from build123d import *

# Parameters (mm, degrees)
CYLINDER002_R     = 0.95
CYLINDER002_DEPTH = 10
CYLINDER003_R     = 0.95
CYLINDER003_DEPTH = 10
CYLINDER_R        = 0.95
CYLINDER_DEPTH    = 10
CYLINDER001_R     = 0.95
CYLINDER001_DEPTH = 10
BOX_W             = 10
BOX_H             = 10
BOX_DEPTH         = 7
PAD_DEPTH         = 21


with BuildPart() as cylinder002:
    # Cylinder002 → Cylinder002 (new body)
    with BuildSketch(Plane(origin=(9.9, 0, 0), x_dir=(1, 0, 0), z_dir=(0, 0, 1))):
        Circle(CYLINDER002_R)
    extrude(amount=CYLINDER002_DEPTH)


with BuildPart() as tornillos001:
    # Cylinder003 → Cylinder003 (new body)
    with BuildSketch(Plane.XY):
        Circle(CYLINDER003_R)
    extrude(amount=CYLINDER003_DEPTH)

    # Fusion001: union Cylinder002
    add(cylinder002.part)


with BuildPart() as tornillos001_1:
    # Fusion001 placement: moved
    add(tornillos001.part.moved(Location((5, -24.5, 22))))


with BuildPart() as cylinder:
    # Cylinder → Cylinder (new body)
    with BuildSketch(Plane(origin=(9.9, 0, 0), x_dir=(1, 0, 0), z_dir=(0, 0, 1))):
        Circle(CYLINDER_R)
    extrude(amount=CYLINDER_DEPTH)


with BuildPart() as fusion002:
    # Cylinder001 → Cylinder001 (new body)
    with BuildSketch(Plane.XY):
        Circle(CYLINDER001_R)
    extrude(amount=CYLINDER001_DEPTH)

    # Fusion: union Cylinder
    add(cylinder.part)


with BuildPart() as fusion002_1:
    # Fusion placement: moved
    add(fusion002.part.moved(Location((5, 24.5, 22))))

    # Fusion002: union Tornillos001
    add(tornillos001_1.part)


with BuildPart() as fusion002_2:
    # Fusion002 placement: moved
    add(fusion002_1.part.moved(Location((0.4, 0, 0))))


with BuildPart() as cube:
    # Box → Box (new body)
    with BuildSketch(Plane(origin=(5, -29, 4), x_dir=(1, 0, 0), z_dir=(0, 0, 1))):
        with Locations((5, 5)):
            Rectangle(BOX_W, BOX_H)
    extrude(amount=BOX_DEPTH)


with BuildPart() as holder001:
    # Sketch → Pad (new body)
    with BuildSketch(Plane.YZ):
        Polygon((-28.75, 32), (-28.75, 0), (28.75, 0), (28.75, 32), (20.75, 32), (20.75, 3.5), (-20.75, 3.5), (-20.75, 32), align=None)
    extrude(amount=PAD_DEPTH)

    # Cut: cut Cube
    add(cube.part, mode=Mode.SUBTRACT)

    # Cut001: cut Fusion002
    add(fusion002_2.part, mode=Mode.SUBTRACT)


solid = holder001.part
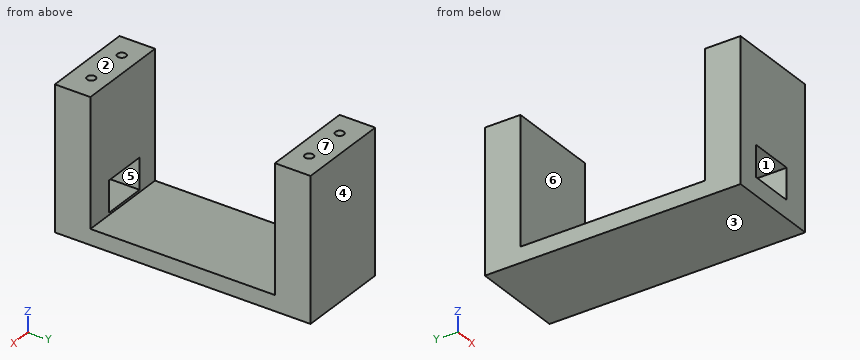
Design review of the part built by this model. Coordinates are the model's own, in mm. Face numbers are marked on the shaded views. A direction names the side the tool comes from. Round coordinates to 2 decimals unless told otherwise and drop trailing zeros. Write each loop counter-clockwise with the first axis right and the second up, starting at its lowest first coordinate (ties: lowest second). Pieces come first, ordered by that corner, then holes. Notation, with made-up numbers: M 57,66.5 L 63,66.5 A24 ccw 63,94.5 Z; hole C 28,14 d6. An arc over 180 degrees is marked long. One line per item, written item: value. Start each with the question number.
1. Take a section at C-C on y = -24.5. State the section outline as (x, z) points, then the cut area to 3 significant figures.
2. Clearance check with flat-ended pins moving along their axes: P1, Ø4, axis at x = 14.5, y = 6, coming from the +Z side; P2, Ø0.9, axis at x = 15.5, y = 24.5, coming from the +Z side. State where each tip first meets the part, or that it passes through.
3. For the marked faces 5, 6 and 7, list the 3-axis set-ups (+Z, -Z, +X, -X, +Y, -Y) from which the entire face can be reached by the end or side of a thin tool; tool diameter is ignored.
4. Take a section at D-D on z = 5. State the section outline as (x, y) points.
5. To check wall thickness, follow probe 1 along Y at (x, z) = (15.3, 26.5); probe 2 along Y at (x, z) = (8.5, 16); probe 3 along X at (y, z) = (-24, 26). State the ranges of each line that lie inside material, in increasing order. Write a range as from..to.
6. Take a section at A-A on x = 12.5. State the section outline as (y, z) points.
7. Take a section at B-B on z = 16.5. State the section outline as (x, y) points.
8. Draft analysis for pull direction Z (two halves, no side actions). For the marked faces 1, 2, 3 and 4, state which applies: pulls with the +Z half, pulls with the -Z half, needs draft (parallel to the pull), parting line crosses it, or undercut.
Computed:
1. outline: M 0,0 L 21,0 L 21,32 L 16.25,32 L 16.25,22 L 14.35,22 L 14.35,32 L 6.35,32 L 6.35,22 L 4.45,22 L 4.45,32 L 0,32 Z; hole M 5,4 L 15,4 L 15,11 L 5,11 Z
1. area: 564 mm²
2. P1: stops at z = 3.5
2. P2: stops at z = 22
3. face 5: -Y
3. face 6: +Z, +X, -X
3. face 7: +Z, +X, -X, +Y, -Y
4. outline: M 0,-28.75 L 5,-28.75 L 5,-20.75 L 0,-20.75 Z; M 0,20.75 L 21,20.75 L 21,28.75 L 0,28.75 Z; M 15,-28.75 L 21,-28.75 L 21,-20.75 L 15,-20.75 Z
5. probe 1: y = -28.75..-25.45, -23.55..-20.75, 20.75..23.55, 25.45..28.75
5. probe 2: y = -28.75..-20.75, 20.75..28.75
5. probe 3: x = 0..4.59, 6.21..14.49, 16.11..21
6. outline: M -28.75,0 L 28.75,0 L 28.75,32 L 20.75,32 L 20.75,3.5 L -20.75,3.5 L -20.75,4 L -28.75,4 Z; M -28.75,11 L -20.75,11 L -20.75,32 L -28.75,32 Z
7. outline: M 0,-28.75 L 21,-28.75 L 21,-20.75 L 0,-20.75 Z; M 0,20.75 L 21,20.75 L 21,28.75 L 0,28.75 Z
8. face 1: undercut
8. face 2: pulls with the +Z half
8. face 3: pulls with the -Z half
8. face 4: needs draft
